```python
from build123d import *

# Parameters (mm, degrees)
EXTRUDE_1_DEPTH = 5


with BuildPart() as part:
    # 草图1 → 凸台-拉伸1 (new body)
    with BuildSketch(Plane(origin=(0, 0, 0), x_dir=(0, 0, -1), z_dir=(1, 0, 0))):
        Polygon((-30.407718659, 7.81238306), (14.592281341, 7.81238306), (14.592281341, 19.81238306), (54.592281341, 19.81238306), (54.592281341, 7.81238306), (79.592281341, 7.81238306), (79.592281341, -0.18761694), (44.592281341, -0.18761694), (44.592281341, 7.81238306), (44.592281341, 11.81238306), (24.592281341, 11.81238306), (24.592281341, 3.81238306), (24.592281341, -0.18761694), (-30.407718659, -0.18761694), align=None)
        with BuildLine():
            Line((-23.407718659, 5.31238306), (-17.407718659, 5.31238306))
            ThreePointArc((-17.407718659, 5.31238306), (-15.907718659, 3.81238306), (-17.407718659, 2.31238306))
            Line((-17.407718659, 2.31238306), (-23.407718659, 2.31238306))
            ThreePointArc((-23.407718659, 2.31238306), (-24.907718659, 3.81238306), (-23.407718659, 5.31238306))
        make_face(mode=Mode.SUBTRACT)
        with BuildLine():
            Line((69.592281341, 2.31238306), (63.592281341, 2.31238306))
            ThreePointArc((63.592281341, 2.31238306), (62.092281341, 3.81238306), (63.592281341, 5.31238306))
            Line((63.592281341, 5.31238306), (69.592281341, 5.31238306))
            ThreePointArc((69.592281341, 5.31238306), (71.092281341, 3.81238306), (69.592281341, 2.31238306))
        make_face(mode=Mode.SUBTRACT)
    extrude(amount=EXTRUDE_1_DEPTH)


solid = part.part
```
Work out the finished part from the listing and answer in its coordinate system (mm). A direction names the side the tool comes from. Give positions to 0.01 mm unless a question says otherwise; leave off trailing zeros. Write each loop counter-clockwise with the first axis right and the second up, starting at its lowest first coordinate (ties: lowest second). Pieces come first, ordered by that corner, then holes.
(1) The part is cut by section A-A on x = 1.15. Write down the section's boundary in (y, z), plus the area to 3 significant figures.
Final values:
outline: (-0.19, -79.59) - (7.81, -79.59) - (7.81, -54.59) - (19.81, -54.59) - (19.81, -14.59) - (7.81, -14.59) - (7.81, 30.41) - (-0.19, 30.41) - (-0.19, -24.59) - (11.81, -24.59) - (11.81, -44.59) - (-0.19, -44.59) - close; hole (2.31, -69.59) arc R1.5 ccw to (5.31, -69.59) - (5.31, -63.59) arc R1.5 ccw to (2.31, -63.59) - close; hole (2.31, 17.41) arc R1.5 ccw to (5.31, 17.41) - (5.31, 23.41) arc R1.5 ccw to (2.31, 23.41) - close
area: 1,070 mm2
(2) Flat-ended cylindrical pins translate along their axes: pin 1 Ø1.5 at (x, y) = (1.5, 13.5) entering from -Z; pin 2 Ø2.5 at (x, z) = (2, 19.5) entering from +Y; pin 3 Ø8 at (y, z) = (5.5, -35) entering from -X. Find the tip coordinate at first contact, or state that the pin passes through.
Final values:
pin 1: stops at z = -54.59
pin 2: stops at y = 7.81
pin 3: passes through
(3) Straight lines are drawn through the part: line 1 (Z direction, x = 1.45, y = 6.5); line 2 (Z direction, x = 0.55, y = 8.25); line 3 (Z direction, x = 0.65, y = 2.75). For each, find the intervals that lie inside material, in ascending order.
Final values:
line 1: z = -79.59 to -44.59, -24.59 to 30.41
line 2: z = -54.59 to -44.59, -24.59 to -14.59
line 3: z = -79.59 to -70.65, -62.53 to -44.59, -24.59 to 16.35, 24.47 to 30.41
(4) The mould has two halves that part along Y. Classify faces 5 (the flat face through (2, 11.812, -35)), 6 (the cylindrical face through (2.46, 3.85, 15.91)), 7 (the flat face through (2, 6, -44.592)): pulls with the +Y half, pulls with the -Y half, needs draft (parallel to the pull), parting line crosses it, or undercut.
Final values:
face 5: pulls with the -Y half
face 6: undercut
face 7: needs draft
(5) The part is cut by section D-D on z = -36. Write down the section's boundary in (x, y).
Final values:
outline: (0, 11.81) - (5, 11.81) - (5, 19.81) - (0, 19.81) - close
(6) The part is cut by section C-C on y = 10. Write down the section's boundary in (x, z).
Final values:
outline: (0, -54.59) - (5, -54.59) - (5, -44.59) - (0, -44.59) - close; (0, -24.59) - (5, -24.59) - (5, -14.59) - (0, -14.59) - close
(7) Which of the six approach directions +Z, -Z, +X, -X, +Y, -Y give full straight-line access (tool end or side, diameter ignored) to faces 1 (the flat face through (2, 6, -24.592)), 2 (the flat face through (2, 7.812, -67)), 3 (the cylindrical face through (2.46, 3.85, -71.09)), 4 (the flat face through (2, 14, -14.592))?
Final values:
face 1: +X, -X, -Y
face 2: -Z, +X, -X, +Y
face 3: +X, -X
face 4: +Z, +X, -X, +Y
(8) The part is cut by section B-B on y = 1. Write down the section's boundary in (x, z).
Final values:
outline: (0, -79.59) - (5, -79.59) - (5, -44.59) - (0, -44.59) - close; (0, -24.59) - (5, -24.59) - (5, 30.41) - (0, 30.41) - close
